Autodesk Inventor part; units mm, degrees
ref_plane "YZ Plane" through (0, 0, 0) normal (1, 0, 0) x (0, 1, 0)
ref_plane "XZ Plane" through (0, 0, 0) normal (0, 1, 0) x (-1, 0, 0)
ref_plane "XY Plane" through (0, 0, 0) normal (0, 0, 1) x (1, 0, 0)
sketch "Sketch1" plane through (0, 0, 0) normal (0, 1, 0) x (-1, 0, 0)
  line L0 (37.5, -37.5) -> (-37.5, -37.5) construction
  line L1 (-37.5, -37.5) -> (-37.5, 37.5) construction
  line L2 (-37.5, 37.5) -> (37.5, 37.5) construction
  line L3 (37.5, 37.5) -> (37.5, -37.5) construction
  circle A0 centre (37.5, -37.5) radius 27 construction
  circle A1 centre (-37.5, -37.5) radius 27 construction
  circle A2 centre (-37.5, 37.5) radius 27 construction
  circle A3 centre (37.5, 37.5) radius 27 construction
  circle A4 centre (37.5, -37.5) radius 27.75
  circle A5 centre (-37.5, -37.5) radius 27.75
  circle A6 centre (-37.5, 37.5) radius 27.75
  circle A7 centre (37.5, 37.5) radius 27.75
  line L4 (75, -75) -> (-75, -75)
  line L5 (-75, -75) -> (-75, 75)
  line L6 (-75, 75) -> (75, 75)
  line L7 (75, 75) -> (75, -75)
  point P0 (0, 0)
  point P1 (-37.5, 0)
  point P2 (0, -37.5)
  point P3 (-75, 0)
  point P4 (0, -75)
  dimension "d0" = 75
  dimension "d1" = 54
  dimension "d2" = 0.75
  dimension "d3" = 0.75
  dimension "d4" = 0.75
  dimension "d5" = 0.75
  dimension "d6" = 150
extrude "Extrusion1" add sketch "Sketch1" along normal blind 3
sketch "Sketch2" plane through (0, 0, 0) normal (0, -1, 0) x (1, 0, 0)
  circle A0 centre (0, 0) radius 7.5
  line L0 (-75, 75) -> (75, 75) construction
  line L1 (-75, -75) -> (-75, 75) construction
  line L2 (75, -75) -> (-75, -75) construction
  line L3 (75, 75) -> (75, -75) construction
  circle A1 centre (-37.5, 37.5) radius 27.75 construction
  circle A2 centre (37.5, 37.5) radius 27.75 construction
  circle A3 centre (37.5, -37.5) radius 27.75 construction
  circle A4 centre (-37.5, -37.5) radius 27.75 construction
  line L4 (66, 66) -> (-66, 66) construction
  line L5 (-66, 66) -> (-66, -66) construction
  line L6 (-66, -66) -> (66, -66) construction
  line L7 (66, -66) -> (66, 66) construction
  circle A5 centre (-66, 66) radius 7.5
  circle A6 centre (66, 66) radius 7.5
  circle A7 centre (-66, -66) radius 7.5
  circle A8 centre (66, -66) radius 7.5
  dimension "d9" = 15
  dimension "d10" = 9
extrude "Extrusion2" add sketch "Sketch2" along normal blind 45
fillet "Fillet1" radius 10 4 edges at (-75, 1.5, 75) (75, 1.5, 75) (75, 1.5, -75) (-75, 1.5, -75)
properties part number "4BeakerStand_3DPrint"
The listing builds one solid part. Answer for the finished solid, in the listing's coordinates (mm). A direction names the side the tool comes from. Give positions to 0.01 mm unless a question says otherwise; leave off trailing zeros. Order: outer loops, then holes, each group sorted by start corner. A loop starts at its lowest first (then second) coordinate and runs counter-clockwise, first axis right, second up. Notation, with made-up numbers: (43.5, 37.5) - (96.5, 37.5) arc R4 cw to (96.5, 41.5) - close; hole circle Ø11 at (-37.75, -37.75). An arc over 180 degrees is marked (long way). Answer in a Markdown table with one row per item. Add a question column.
Q1. The part is cut by section C-C (x = 0). Determine the outline of the cut face in (y, z), then the cut area to 4 significant figures.
Q2. The part is cut by section B-B (x = -37.5). Determine the outline of the cut face in (y, z), then the cut area to 3 significant figures.
Q3. The part is cut by section A-A (z = 37.5). Determine the outline of the cut face in (x, y), then the cut area to 3 significant figures.
Q4. Which of the six approach directions +Z, -Z, +X, -X, +Y, -Y give full straight-line access (tool end or side, diameter ignored) to faces 5 (the cylindrical face through (11.031, 1.479, 29.165)), 6 (the flat face through (1, 0, 18))?
Q5. Find the intervals of material crossed by line 1 along Z through (x, y) = (-37, 1); line 2 along Y through (x, z) = (4, 30), in increasing order. Write a range as [from, to].
Q6. For a pull along Z with two mould halves and no side action, classify faces 1 (the cylindrical face through (-71.99, 1.52, -72.15)), 2 (the cylindrical face through (-7.493, -22.185, -0.33)), 3 (the cylindrical face through (-66.976, -22.185, 58.564)), 4 (the flat face through (-66, -45, -66)) as released by +Z, released by -Z, zero draft, split by the parting line, or undercut.
Q7. Given P1, Ø2, axis at x = 5, z = 15, coming from the -Y side; P2, Ø12, axis at y = -18.5, z = 6, coming from the +X side, each flat-ended and moving along its own axis, determine where each tip first touches the part or whether it passes through.
Q8. The part is cut by section D-D (z = 0). Determine the outline of the cut face in (x, y).
Determined:
| question | item | result |
|---|---|---|
| 1 | outline | (-45, -7.5) - (0, -7.5) - (0, -75) - (3, -75) - (3, 75) - (0, 75) - (0, 7.5) - (-45, 7.5) - close |
| 1 | area | 1,125 mm² |
| 2 | outline | (0, -75) - (3, -75) - (3, -65.25) - (0, -65.25) - close; (0, -9.75) - (3, -9.75) - (3, 9.75) - (0, 9.75) - close; (0, 65.25) - (3, 65.25) - (3, 75) - (0, 75) - close |
| 2 | area | 117 mm² |
| 3 | outline | (-75, 0) - (-65.25, 0) - (-65.25, 3) - (-75, 3) - close; (-9.75, 0) - (9.75, 0) - (9.75, 3) - (-9.75, 3) - close; (65.25, 0) - (75, 0) - (75, 3) - (65.25, 3) - close |
| 3 | area | 117 mm² |
| 4 | face 5 | +Y, -Y |
| 4 | face 6 | -Y |
| 5 | line 1 | z = [-75, -65.25], [-9.75, 9.75], [65.25, 75] |
| 5 | line 2 | y = [0, 3] |
| 6 | face 1 | released by -Z |
| 6 | face 2 | split by the parting line |
| 6 | face 3 | undercut |
| 6 | face 4 | zero draft |
| 7 | P1 | stops at y = 0 |
| 7 | P2 | stops at x = 7.5 |
| 8 | outline | (-75, 0) - (-7.5, 0) - (-7.5, -45) - (7.5, -45) - (7.5, 0) - (75, 0) - (75, 3) - (-75, 3) - close |
